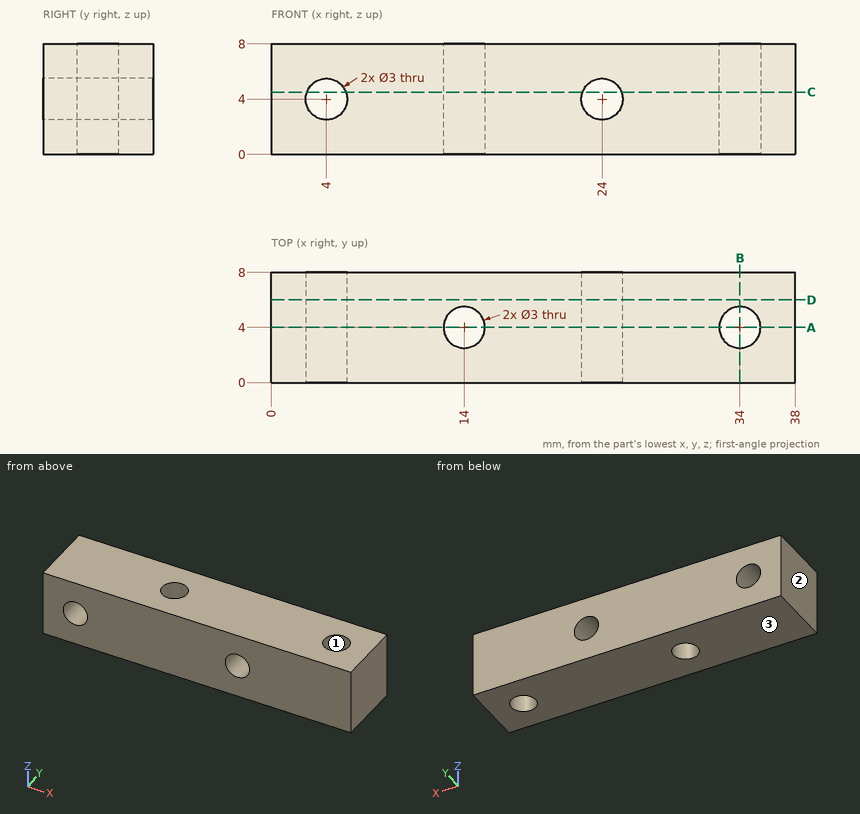
Verification items for this drawing (mm, ordinates from the low corner). Coordinates: 2 decimals unless noted, no trailing zeros. Loops run counter-clockwise (first coordinate to the right, second up) from the corner with the lowest first, then second, coordinate; pieces in that order, holes last. Notation, with made-up numbers: (25, 30.25) - (61, 30.25) arc R20 cw to (61, 53.25) - close; hole circle Ø5 at (-19.75, 63). An arc over 180 degrees is marked (long way). Answer as a JSON object with one key per item and string values.
(1) Cross-section at A-A, the plane y = 4. Record the boundary of the cut face in (x, z), then the cut area to 3 significant figures.
Response:
{"outline": "(0, 0) - (12.5, 0) - (12.5, 8) - (0, 8) - close; (15.5, 0) - (32.5, 0) - (32.5, 8) - (15.5, 8) - close; (35.5, 0) - (38, 0) - (38, 8) - (35.5, 8) - close; hole circle Ø3 at (4, 4); hole circle Ø3 at (24, 4)", "area": "242 mm²"}
(2) Go/stop test with a flat-tipped pin: pin 1 Ø1.8 at (x, z) = (4, 4) entering from +Y. Record where the tip stops, or that it passes through.
Response:
{"pin 1": "passes through"}
(3) Cross-section at B-B, the plane x = 34. Record the boundary of the cut face in (y, z).
Response:
{"outline": "(0, 0) - (2.5, 0) - (2.5, 8) - (0, 8) - close; (5.5, 0) - (8, 0) - (8, 8) - (5.5, 8) - close"}
(4) Scan lines: line 1 along X through (y, z) = (5.75, 4); line 2 along Z through (x, y) = (4, 4). Record each from-to range of solid material in increasing order.
Response:
{"line 1": "x = 0 to 2.5, 5.5 to 22.5, 25.5 to 38", "line 2": "z = 0 to 2.5, 5.5 to 8"}
(5) Mould release check, pull along X, two halves, no side actions. Record for the marked faces 1, 2 and 3: pulls with the +X half, pulls with the -X half, needs draft (parallel to the pull), parting line crosses it, or undercut.
Response:
{"face 1": "undercut", "face 2": "pulls with the -X half", "face 3": "needs draft"}
(6) Cross-section at D-D, the plane y = 6. Record the boundary of the cut face in (x, z).
Response:
{"outline": "(0, 0) - (38, 0) - (38, 8) - (0, 8) - close; hole circle Ø3 at (4, 4); hole circle Ø3 at (24, 4)"}
(7) Cross-section at C-C, the plane z = 4.5. Record the boundary of the cut face in (x, y).
Response:
{"outline": "(0, 0) - (2.59, 0) - (2.59, 8) - (0, 8) - close; (5.41, 0) - (22.59, 0) - (22.59, 8) - (5.41, 8) - close; (25.41, 0) - (38, 0) - (38, 8) - (25.41, 8) - close; hole circle Ø3 at (14, 4); hole circle Ø3 at (34, 4)"}
